Read the model definition and answer for the solid it produces. Units are mm, in the model's axes. Coordinates: 2 decimals unless noted, no trailing zeros. Write each loop counter-clockwise with the first axis right and the second up, starting at its lowest first coordinate (ties: lowest second). Pieces come first, ordered by that corner, then holes.
1) Determine the mould class of faces 1 (the face through (0, 19, 0.508)), 2 (the face through (-0.355, 44.617, 0.258)) for opening direction Y: +Y half, -Y half, draft (parallel to the pull), parting line (faces both ways), or undercut.
2) The part is cut by section D-D (x = -13.5). Determine the outline of the cut face in (y, z) (3 decimals).
3) Find the intervals of material crossed by line 1 (Y direction, x = 0, z = 0.1); line 2 (X direction, y = 42, z = 0.1); line 3 (X direction, y = 24, z = 0.4), in increasing order.
4) The part is cut by section C-C (y = 30.5). Determine the outline of the cut face in (x, z), then the cut area to 3 significant figures.
5) The part is cut by section B-B (x = 2). Determine the outline of the cut face in (y, z), then the cut area to 3 significant figures.
from build123d import *

# Parameters (mm, degrees)
F1_DEPTH = 0.508
F2_R     = 2.7305
F3_DEPTH = 0.509
F4_R     = 0.508


with BuildPart() as f1:
    # F0 (on Top) → F1 (new body)
    with BuildSketch(Plane.XY):
        with BuildLine():
            Line((-15.875, 0), (0, 0))
            Line((0, 0), (15.875, 0))
            Line((15.875, 0), (15.875, 6.985))
            Line((15.875, 6.985), (6.35, 6.985))
            Line((6.35, 6.985), (6.35, 41.91))
            ThreePointArc((6.35, 41.91), (4.490128, 46.400128), (0, 48.26))
            ThreePointArc((0, 48.26), (-4.490128, 46.400128), (-6.35, 41.91))
            Line((-6.35, 41.91), (-6.35, 6.985))
            Line((-6.35, 6.985), (-15.875, 6.985))
            Line((-15.875, 6.985), (-15.875, 0))
        make_face()
    extrude(amount=F1_DEPTH)

    # F2 (on face) → F3 (cut, through all)
    with BuildSketch(Plane.XY.offset(0.508)):
        with Locations((0, 41.91)):
            Circle(F2_R)
    extrude(amount=-F3_DEPTH, mode=Mode.SUBTRACT)

    # F4
    f4_edges = [f1.edges().sort_by_distance(p)[0] for p in [
        (-15.875, 0, 0.254),
        (-15.875, 6.985, 0.254),
        (15.875, 6.985, 0.254),
        (15.875, 0, 0.254),
        (6.35, 6.985, 0.254),
        (-6.35, 6.985, 0.254),
    ]]
    fillet(f4_edges, radius=F4_R)


solid = f1.part
Reported:
1. face 1: draft
1. face 2: undercut
2. outline: (0, 0) - (6.985, 0) - (6.985, 0.508) - (0, 0.508) - close
3. line 1: y = 0 to 39.18, 44.64 to 48.26
3. line 2: x = -6.35 to -2.73, 2.73 to 6.35
3. line 3: x = -6.35 to 6.35
4. outline: (-6.35, 0) - (6.35, 0) - (6.35, 0.51) - (-6.35, 0.51) - close
4. area: 6.45 mm2
5. outline: (0, 0) - (40.05, 0) - (40.05, 0.51) - (0, 0.51) - close; (43.77, 0) - (47.94, 0) - (47.94, 0.51) - (43.77, 0.51) - close
5. area: 22.5 mm2
